Check sheet for the modelled part. Datum: model origin and axes. Units: mm. A direction names the side the tool comes from. Round coordinates to 2 decimals unless told otherwise and drop trailing zeros. Loops run counter-clockwise (first coordinate to the right, second up) from the corner with the lowest first, then second, coordinate; pieces in that order, holes last. Notation, with made-up numbers: (-18.75, 49) - (-10.75, 49) arc R18 cw to (-10.75, 72) - close; hole circle Ø9 at (62, -6.5). An arc over 180 degrees is marked (long way). Return JSON: item names as keys, results as strings.
from build123d import *

# Parameters (mm, degrees)
SKETCH1_W           = 68.58
SKETCH1_H           = 68.58
SKETCH1_W_2         = 60.58
SKETCH1_H_2         = 60.58
BOSS_EXTRUDE1_DEPTH = 25.4
SKETCH2_R           = 73.025
BOSS_EXTRUDE2_DEPTH = 6.35


with BuildPart() as part:
    # Sketch1 → Boss-Extrude1 (new body)
    with BuildSketch(Plane(origin=(0, 0, 0), x_dir=(1, 0, 0), z_dir=(0, 1, 0))):
        Rectangle(SKETCH1_W, SKETCH1_H)
        Rectangle(SKETCH1_W_2, SKETCH1_H_2, mode=Mode.SUBTRACT)
    extrude(amount=BOSS_EXTRUDE1_DEPTH)

    # Sketch2 → Boss-Extrude2 (add)
    with BuildSketch(Plane(origin=(0, 0, 0), x_dir=(1, 0, 0), z_dir=(0, 1, 0))):
        Circle(SKETCH2_R)
    extrude(amount=BOSS_EXTRUDE2_DEPTH)


solid = part.part
Q1. Scan lines: probe 1 along Z at (x, y) = (-23, 14); probe 2 along X at (y, z) = (23.75, -31). Record each from-to range of solid material in increasing order. Write a range as [from, to].
Answer key:
{"probe 1": "z = [-34.29, -30.29], [30.29, 34.29]", "probe 2": "x = [-34.29, 34.29]"}
Q2. Sectioned sample at C-C (z = 0). Enter the section's corners in (x, y) (3 decimals).
Answer key:
{"outline": "(-73.025, 0) - (73.025, 0) - (73.025, 6.35) - (34.29, 6.35) - (34.29, 25.4) - (30.29, 25.4) - (30.29, 6.35) - (-30.29, 6.35) - (-30.29, 25.4) - (-34.29, 25.4) - (-34.29, 6.35) - (-73.025, 6.35) - close"}
Q3. Depth check by flat-ended pin: P1, Ø15, axis at y = 20.5, z = 10.5, coming from the -X side; P2, Ø6, axis at x = -1, z = -26, coming from the +Y side; P3, Ø1.5, axis at y = 6.5, z = 9, coming from the -X side. Enter the tip coordinate at first touch or a pass-through.
Answer key:
{"P1": "stops at x = -34.29", "P2": "stops at y = 6.35", "P3": "stops at x = -72.56"}
Q4. Sectioned sample at A-A (y = 22.75). Enter the section's corners in (x, z).
Answer key:
{"outline": "(-34.29, -34.29) - (34.29, -34.29) - (34.29, 34.29) - (-34.29, 34.29) - close; hole (-30.29, -30.29) - (30.29, -30.29) - (30.29, 30.29) - (-30.29, 30.29) - close"}
Q5. Sectioned sample at D-D (y = 2). Enter the section's corners in (x, z) (3 decimals).
Answer key:
{"outline": "circle Ø146.05 at (0, 0)"}
Q6. Tool access check on faces 5 (the face through (-30.29, 16, 0)), 6 (the face through (-31, 25.4, 0)), 7 (the face through (0, 16, -34.29)), 8 (the face through (-34.29, 16, 0)). Record the directions out of +Z, -Z, +X, -X, +Y, -Y that give a thin tool (end or side, any length) a straight path to the whole face; none if there is none.
Answer key:
{"face 5": "+Y", "face 6": "+Z, -Z, +X, -X, +Y", "face 7": "-Z, +X, -X, +Y", "face 8": "+Z, -Z, -X, +Y"}
Q7. Sectioned sample at B-B (x = 0). Enter the section's corners in (y, z) (3 decimals).
Answer key:
{"outline": "(0, -73.025) - (6.35, -73.025) - (6.35, -34.29) - (25.4, -34.29) - (25.4, -30.29) - (6.35, -30.29) - (6.35, 30.29) - (25.4, 30.29) - (25.4, 34.29) - (6.35, 34.29) - (6.35, 73.025) - (0, 73.025) - close"}
Q8. Draft check along X on faces 1 (the face through (0, 16, 34.29)), 2 (the face through (69.653, 3.131, -21.935)), 3 (the face through (34.29, 16, 0)), 4 (the face through (0, 16, -30.29)). Enter one of: released by +X, released by -X, zero draft, split by the parting line, or undercut.
Answer key:
{"face 1": "zero draft", "face 2": "split by the parting line", "face 3": "released by +X", "face 4": "undercut"}
